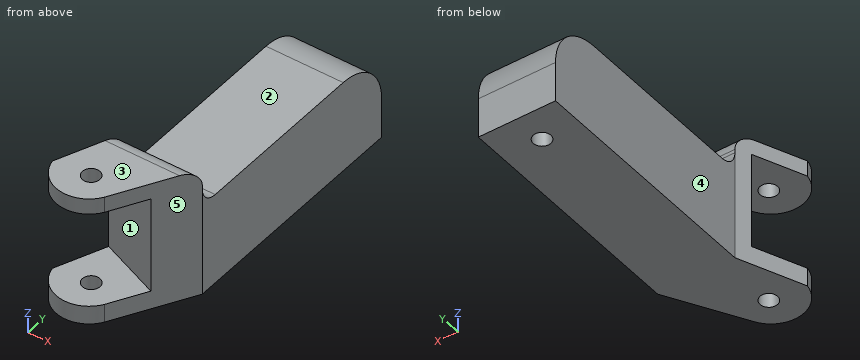
```python
from build123d import *

# Parameters (mm, degrees)
EXTRUDE_1_DEPTH     = 53
EXTRUDE_2_DEPTH     = 22
FILLET_2_R          = 10
FILLET_3_R          = 10
SKETCH_3_W          = 55.304366744
SKETCH_3_H          = 61.895042574
CUT_EXTRUDE_1_DEPTH = 56
SKETCH_4_R          = 5
CUT_EXTRUDE_2_DEPTH = 75
SKETCH_5_R          = 5
CUT_EXTRUDE_3_DEPTH = 10
FILLET_4_R          = 30


with BuildPart() as part:
    # Эскиз1 → Бобышка-Вытянуть1 (new body)
    with BuildSketch(Plane.XY):
        with BuildLine():
            Line((7.580184654, -59.799234496), (-16.79145183, -102.52734615))
            ThreePointArc((-16.79145183, -102.52734615), (-36.438294134, -111.229048288), (-51.465460174, -95.869936548))
            Line((-51.465460174, -95.869936548), (-36.497185373, -59.799234496))
            Line((-36.497185373, -59.799234496), (-36.497185373, 79.732312661))
            Line((-36.497185373, 79.732312661), (7.580184654, 79.732312661))
            Line((7.580184654, 79.732312661), (7.580184654, -59.799234496))
        make_face()
    extrude(amount=EXTRUDE_1_DEPTH)

    # Эскиз2 → Бобышка-Вытянуть2 (add)
    with BuildSketch(Plane.XY.offset(53)):
        with BuildLine():
            Line((-36.497185373, -59.799234496), (7.580184654, -59.799234496))
            Line((7.580184654, -59.799234496), (-16.79145183, -102.52734615))
            ThreePointArc((-16.79145183, -102.52734615), (-36.438294134, -111.229048288), (-51.465460174, -95.869936548))
            Line((-51.465460174, -95.869936548), (-36.497185373, -59.799234496))
        make_face()
    extrude(amount=EXTRUDE_2_DEPTH)

    # Скругление2
    fillet_2_edges = [part.edges().sort_by_distance(p)[0] for p in [
        (-14.458500359, -59.799234496, 53),
    ]]
    fillet(fillet_2_edges, radius=FILLET_2_R)

    # Скругление3
    fillet_3_edges = [part.edges().sort_by_distance(p)[0] for p in [
        (-14.458500359, -59.799234496, 75),
    ]]
    fillet(fillet_3_edges, radius=FILLET_3_R)

    # Эскиз3 → Вырез-Вытянуть1 (cut)
    with BuildSketch(Plane(origin=(-9.966103605, 4.135638315, 0), x_dir=(0, 0, 1), z_dir=(-0.923632182, 0.383280045, 0))):
        with Locations((38.275019494, -109.025889751)):
            Rectangle(SKETCH_3_W, SKETCH_3_H)
    extrude(amount=-CUT_EXTRUDE_1_DEPTH, mode=Mode.SUBTRACT)

    # Эскиз4 → Вырез-Вытянуть2 (cut)
    with BuildSketch(Plane.XY.offset(75)):
        with Locations((-31.007416938, -93.698436978)):
            Circle(SKETCH_4_R)
    extrude(amount=-CUT_EXTRUDE_2_DEPTH, mode=Mode.SUBTRACT)

    # Эскиз5 → Вырез-Вытянуть3 (cut)
    with BuildSketch(Plane(origin=(0, 0, 0), x_dir=(-1, 0, 0), z_dir=(0, 0, -1))):
        with Locations((15.173432646, 61.131642173)):
            Circle(SKETCH_5_R)
    extrude(amount=-CUT_EXTRUDE_3_DEPTH, mode=Mode.SUBTRACT)

    # Скругление4
    fillet_4_edges = [part.edges().sort_by_distance(p)[0] for p in [
        (-14.458500359, 79.732312661, 53),
    ]]
    fillet(fillet_4_edges, radius=FILLET_4_R)


solid = part.part
```
Read the model definition and answer for the solid it produces. Units are mm, in the model's axes. Face numbers are marked on the shaded views. A direction names the side the tool comes from. Give positions to 0.01 mm unless a question says otherwise; leave off trailing zeros. Loops run counter-clockwise (first coordinate to the right, second up) from the corner with the lowest first, then second, coordinate; pieces in that order, holes last.
Item 1: The part is cut by section A-A (x = -45). Write down the section's boundary in (y, z).
Item 2: For the marked faces 1, 2, 3, 4 and 5, determine the directions among +Z, -Z, +X, -X, +Y, -Y from which every point of the face is accessible in a straight line to the end or side of a thin tool.
Item 3: Each of these flat-tipped pins is pushed along its axis until it touches: pin 1 Ø5 at (x, z) = (-27, 8.5) entering from -Y; pin 2 Ø6 at (x, y) = (-31.01, -93.7) entering from -Z; pin 3 Ø2 at (x, z) = (-14.5, 64) entering from +Y; pin 4 Ø1 at (x, y) = (-2, 8) entering from +Z. Where does it stop, or does it pass through?
Item 4: Find the intervals of material crossed by line 1 along Z through (x, y) = (-44, -88.5); line 2 along Z through (x, y) = (-8, -50); line 3 along X through (y, z) = (43, 12), in increasing order.
Item 5: The part is cut by section C-C (x = -29). Write down the section's boundary in (y, z).
Item 6: The part is cut by section D-D (y = -27.5). Write down the section's boundary in (x, z), and give its area (3 significant figures).
Item 7: The part is cut by section B-B (z = 69). Write down the section's boundary in (x, y), and give its area (3 significant figures).
Taken from the geometry:
1. outline: (-107.16, 0) - (-80.29, 0) - (-80.29, 10.62) - (-107.16, 10.62) - close; (-107.16, 65.93) - (-80.29, 65.93) - (-80.29, 75) - (-107.16, 75) - close
2. face 1: -X, -Y
2. face 2: +Z, +X, -X, +Y
2. face 3: +Z, +X, -X, +Y, -Y
2. face 4: +Z, -Z, -X, +Y
2. face 5: +Z, -Z, +X, -Y
3. pin 1: stops at y = -111.26
3. pin 2: passes through
3. pin 3: stops at y = -59.8
3. pin 4: stops at z = 53
4. line 1: z = 0 to 10.62, 65.93 to 75
4. line 2: z = 0 to 53
4. line 3: x = -36.5 to 7.58
5. outline: (-111.16, 0) - (-98.28, 0) - (-98.28, 10.62) - (-111.16, 10.62) - close; (-111.16, 65.93) - (-98.28, 65.93) - (-98.28, 75) - (-111.16, 75) - close; (-89.12, 0) - (79.73, 0) - (79.73, 23) arc R30 ccw to (49.73, 53) - (-49.8, 53) arc R10 cw to (-59.8, 63) - (-59.8, 65) arc R10 ccw to (-69.8, 75) - (-89.12, 75) - (-89.12, 65.93) - (-72.5, 65.93) - (-72.5, 10.62) - (-89.12, 10.62) - close
6. outline: (-36.5, 0) - (7.58, 0) - (7.58, 53) - (-36.5, 53) - close
6. area: 2,340 mm2
7. outline: (-51.47, -95.87) arc R18.85 ccw to (-16.79, -102.53) - (7.1, -60.63) - (-36.84, -60.63) - close; hole circle Ø10 at (-31.01, -93.7)
7. area: 1,820 mm2
